The model under review builds one solid part; all positions refer to its coordinate system, in mm. Round coordinates to 2 decimals unless told otherwise and drop trailing zeros. Order: outer loops, then holes, each group sorted by start corner. A loop starts at its lowest first (then second) coordinate and runs counter-clockwise, first axis right, second up. Notation, with made-up numbers: M 4.5,82 L 12.5,82 A19 ccw 12.5,98 Z; hole C 21,22.25 d10. An arc over 180 degrees is marked long. One line per item, written item: value. Start each with the question number.
from build123d import *

# Parameters (mm, degrees)
F1_DEPTH = 63.5
F2_W     = 12.7
F2_H     = 190.5
F4_DEPTH = 0.254
F3_W     = 12.7
F3_H     = 190.5
F5_DEPTH = 0.254


with BuildPart() as f1:
    # F0 (on Top) → F1 (new body)
    with BuildSketch(Plane.XY):
        with BuildLine():
            ThreePointArc((19.05, 12.7), (17.190128, 17.190128), (12.7, 19.05))
            Line((12.7, 19.05), (-12.7, 19.05))
            ThreePointArc((-12.7, 19.05), (-17.190128, 17.190128), (-19.05, 12.7))
            Line((-19.05, 12.7), (-19.05, -12.7))
            ThreePointArc((-19.05, -12.7), (-17.190128, -17.190128), (-12.7, -19.05))
            Line((-12.7, -19.05), (12.7, -19.05))
            ThreePointArc((12.7, -19.05), (17.190128, -17.190128), (19.05, -12.7))
            Line((19.05, -12.7), (19.05, 12.7))
        make_face()
    extrude(amount=F1_DEPTH)


with BuildPart() as f4:
    # F2 (on Right) → F4 (new body)
    with BuildSketch(Plane.YZ):
        with Locations((-192.550282, 22.601065)):
            Rectangle(F2_W, F2_H)
    extrude(amount=F4_DEPTH)


with BuildPart() as f5:
    # F3 (on Right) → F5 (new body)
    with BuildSketch(Plane.YZ):
        with Locations((175.864179, 24.777815)):
            Rectangle(F3_W, F3_H)
    extrude(amount=F5_DEPTH)


solid = f1.part
Item 1: Consider section A-A, the plane z = 21.5. Give the boundary of the cut face in (x, y), then the cut area to 3 significant figures.
Item 2: Wall thickness on L1, parallel to X at y = -16.5, z = 51.5; L2, parallel to Y at x = -16, z = 58.5; L3, parallel to Y at x = 14, z = 39: over which ranges is each line inside the solid? List them lowest first.
Item 3: Consider section B-B, the plane y = 16.5. Give the boundary of the cut face in (x, z).
Item 4: Consider section C-C, the plane y = -16. Give the boundary of the cut face in (x, z), then the cut area to 3 significant figures.
Computed:
1. outline: M -19.05,-12.7 A6.35 ccw -12.7,-19.05 L 12.7,-19.05 A6.35 ccw 19.05,-12.7 L 19.05,12.7 A6.35 ccw 12.7,19.05 L -12.7,19.05 A6.35 ccw -19.05,12.7 Z
1. area: 1,420 mm^2
2. L1: x = -17.79 to 17.79
2. L2: y = -18.13 to 18.13
2. L3: y = -18.92 to 18.92
3. outline: M -17.79,0 L 17.79,0 L 17.79,63.5 L -17.79,63.5 Z
4. outline: M -18.13,0 L 18.13,0 L 18.13,63.5 L -18.13,63.5 Z
4. area: 2,300 mm^2
